Check sheet for the modelled part. Datum: model origin and axes. Units: mm. A direction names the side the tool comes from. Give positions to 0.01 mm unless a question says otherwise; leave off trailing zeros. Loops run counter-clockwise (first coordinate to the right, second up) from the corner with the lowest first, then second, coordinate; pieces in that order, holes last. Notation, with made-up numbers: (58, 14) - (75, 14) arc R36 cw to (75, 48) - close; hole circle Ø7 at (71.5, 79.5). An arc over 180 degrees is marked (long way). Answer in a Markdown table with one row per item. Add a question column.
(1) Sectioned sample at B-B on x = 0. Enter the section's corners in (y, z), then the cut area to 3 significant figures.
(2) Thickness scan on L1, parallel to Y at x = -0.25, z = -0.5; L2, parallel to Y at x = -3, z = 4.5; L3, parallel to X at y = -7.5, z = -1.5. Record the ranges inside material, lowest first.
(3) Sectioned sample at C-C on y = -12.25. Enter the section's corners in (x, z).
(4) Go/stop test with flat-tipped pins: P1, Ø2.5, axis at x = -1, z = 7, coming from the -Y side; P2, Ø3.5, axis at y = -1, z = 4, coming from the -X side; P3, Ø4.5, axis at x = 0, z = 1, coming from the -Y side. Record where each tip stops, or that it passes through.
(5) Set-up check for faces 1 (the face through (0, -7.4, -2)), 2 (the face through (0.1, -8.3, 10.3)), 3 (the face through (3, -14, 2)), 4 (the face through (0, -13.6, 2)): record each of +Z, -Z, +X, -X, +Y, -Y from which the full face is reachable in a straight line by a thin tool's end or side.
(6) Draft check along Y on faces 5 (the face through (0, 0, 6)), 6 (the face through (-4.507, -8, 3)), 7 (the face through (0, -7.6, -2)), 8 (the face through (0, -13.8, 7)). Enter one of: released by +Y, released by -Y, zero draft, split by the parting line, or undercut.
from build123d import *

# Parameters (mm, degrees)
SKETCH_W     = 9
SKETCH_H     = 11
PAD_DEPTH    = 3.4
PAD001_DEPTH = 10
FILLET_R     = 0.5
SKETCH002_W  = 2
SKETCH002_H  = 2
PAD002_DEPTH = 0.8
PAD003_DEPTH = 0.2
SKETCH004_R  = 1.4
PAD004_DEPTH = 0.2
PAD005_DEPTH = 0.2


with BuildPart() as part:
    # Sketch → Pad (new body)
    with BuildSketch(Plane.XZ):
        with Locations((0, 5.5)):
            Rectangle(SKETCH_W, SKETCH_H)
    extrude(amount=PAD_DEPTH)

    # Sketch001 (on Face6 of Pad) → Pad001 (join)
    with BuildSketch(Plane.XZ.offset(3.4)):
        with BuildLine():
            ThreePointArc((4, 6.3), (0, 10.3), (-4, 6.3))
            Line((-4, 6.3), (-4.507423, 6.3))
            Line((-4.507423, 6.3), (-4.507423, 0))
            Line((-4.507423, 0), (4.492577, 0))
            Line((4.492577, 0), (4.492577, 6.3))
            Line((4.492577, 6.3), (4, 6.3))
        make_face()
    extrude(amount=PAD001_DEPTH)

    # Fillet
    fillet_edges = [part.edges().sort_by_distance(p)[0] for p in [
        (4.5, -1.7, 11),
        (-4.5, -1.7, 11),
    ]]
    fillet(fillet_edges, radius=FILLET_R)

    # Sketch002 (on Face16 of Fillet) → Pad002 (join)
    with BuildSketch(Plane.XZ.offset(13.4)):
        with Locations((3.5, 1)):
            Rectangle(SKETCH002_W, SKETCH002_H)
        with Locations((-3.5, 1)):
            Rectangle(SKETCH002_W, SKETCH002_H)
    extrude(amount=PAD002_DEPTH)

    # Sketch003 (on Face16 of Pad002) → Pad003 (join)
    with BuildSketch(Plane.XZ.offset(13.4)):
        with BuildLine():
            Line((-1.2, -2.5), (-1.2, 4.9))
            ThreePointArc((1.2, 4.9), (0, 8.5), (-1.2, 4.9))
            Line((1.2, -2.5), (1.2, 4.9))
            ThreePointArc((-1.2, -2.5), (0, -3.699991), (1.2, -2.5))
        make_face()
    extrude(amount=PAD003_DEPTH)

    # Sketch004 (on Face33 of Pad003) → Pad004 (join)
    with BuildSketch(Plane.XZ.offset(13.6)):
        with Locations((0, 6.5)):
            Circle(SKETCH004_R)
    extrude(amount=PAD004_DEPTH)

    # Sketch005 (on DatumPlane) → Pad005 (join)
    with BuildSketch(Plane(origin=(0, -7.4, 0), x_dir=(-1, 0, 0), z_dir=(0, 1, 0))):
        with BuildLine():
            Line((-1.2, 0), (1.2, 0))
            Line((1.2, 0), (1.2, -2.5))
            ThreePointArc((-1.2, -2.5), (0, -3.7), (1.2, -2.5))
            Line((-1.2, 0), (-1.2, -2.5))
        make_face()
    extrude(amount=-PAD005_DEPTH)


solid = part.part
Reply:
| question | item | result |
|---|---|---|
| 1 | outline | (-13.8, 5.1) - (-13.6, 5.1) - (-13.6, -3.7) - (-13.4, -3.7) - (-13.4, 0) - (-7.6, 0) - (-7.6, -3.7) - (-7.4, -3.7) - (-7.4, 0) - (0, 0) - (0, 11) - (-3.4, 11) - (-3.4, 10.3) - (-13.4, 10.3) - (-13.4, 8.5) - (-13.6, 8.5) - (-13.6, 7.9) - (-13.8, 7.9) - close |
| 1 | area | 144 mm^2 |
| 2 | L1 | -13.6 to -13.4, -7.6 to -7.4 |
| 2 | L2 | -13.4 to 0 |
| 2 | L3 | -1.2 to 1.2 |
| 3 | outline | (-4.51, 0) - (4.49, 0) - (4.49, 6.3) - (4, 6.3) arc R4 ccw to (-4, 6.3) - (-4.51, 6.3) - close |
| 4 | P1 | y = -13.8 |
| 4 | P2 | x = -4.5 |
| 4 | P3 | y = -13.6 |
| 5 | face 1 | -Z, +X, -X, +Y |
| 5 | face 2 | +Z, -Y |
| 5 | face 3 | +Z, +X, -Y |
| 5 | face 4 | -Y |
| 6 | face 5 | released by +Y |
| 6 | face 6 | zero draft |
| 6 | face 7 | undercut |
| 6 | face 8 | released by -Y |
